```python
from build123d import *

# Parameters (mm, degrees)
ESBO_O4_R                = 3.5
ESBO_O4_R_2              = 1.5
RESSALTO_EXTRUS_O1_DEPTH = 3


with BuildPart() as part:
    # Esboço4 → Ressalto-extrusão1 (new body)
    with BuildSketch(Plane(origin=(0, 0, 0), x_dir=(1, 0, 0), z_dir=(0, 1, 0))):
        with BuildLine():
            Line((-11.987372598, 93.966613318), (-11.987372598, 71.466613318))
            Line((-11.987372598, 71.466613318), (-11.987372598, -8.633386682))
            ThreePointArc((-11.987372598, -8.633386682), (0.012627402, -20.633386682), (12.012627402, -8.633386682))
            Line((12.012627402, -8.633386682), (12.012627402, 71.466613318))
            Line((12.012627402, 71.466613318), (12.012627402, 93.966613318))
            ThreePointArc((12.012627402, 93.966613318), (9.083695214, 101.03768113), (2.012627402, 103.966613318))
            Line((2.012627402, 103.966613318), (0.012627402, 103.966613318))
            Line((0.012627402, 103.966613318), (-1.987372598, 103.966613318))
            ThreePointArc((-1.987372598, 103.966613318), (-9.05844041, 101.03768113), (-11.987372598, 93.966613318))
        make_face()
        Polygon((0.512627402, -17.633386682), (0.012627402, -17.633386682), (-0.487372598, -17.633386682), (-0.487372598, -11.633386682), (0.512627402, -11.633386682), align=None, mode=Mode.SUBTRACT)
        with Locations(Location((0.012627402, -2.633386682, 0), (0, 0, 270))):
            Circle(ESBO_O4_R, mode=Mode.SUBTRACT)
        Polygon((0.012627402, 12.366613318), (0.512627402, 12.366613318), (0.512627402, 6.366613318), (-0.487372598, 6.366613318), (-0.487372598, 12.366613318), align=None, mode=Mode.SUBTRACT)
        with Locations(Location((0.012627402, 67.966742295, 0), (0, 0, 270))):
            Circle(ESBO_O4_R_2, mode=Mode.SUBTRACT)
        Polygon((6.012627402, 94.466613318), (6.012627402, 71.466613318), (2.487372598, 71.466613318), (-2.487372598, 71.466613318), (-5.987372598, 71.466613318), (-5.987372598, 82.966613318), (-5.987372598, 94.466613318), (-2.5, 94.466613318), (2.5, 94.466613318), align=None, mode=Mode.SUBTRACT)
        with Locations(Location((0.012627402, 97.966613318, 0), (0, 0, 270))):
            Circle(ESBO_O4_R_2, mode=Mode.SUBTRACT)
    extrude(amount=RESSALTO_EXTRUS_O1_DEPTH)


solid = part.part
```
The model under review builds one solid part; all positions refer to its coordinate system, in mm. A direction names the side the tool comes from. Give positions to 0.01 mm unless a question says otherwise; leave off trailing zeros. Write each loop counter-clockwise with the first axis right and the second up, starting at its lowest first coordinate (ties: lowest second). Pieces come first, ordered by that corner, then holes. Notation, with made-up numbers: (-15.5, 44.25) -> (-7.5, 44.25) arc R20 ccw to (-7.5, 70.25) -> close; hole circle Ø1 at (89, 51). An arc over 180 degrees is marked (long way). Put each result on its own line as item: value.
(1) We need section C-C, the plane z = -81. Give the boundary of the cut face in (x, y).
Results are:
outline: (-11.99, 0) -> (-5.99, 0) -> (-5.99, 3) -> (-11.99, 3) -> close; (6.01, 0) -> (12.01, 0) -> (12.01, 3) -> (6.01, 3) -> close
(2) We need section A-A, the plane z = -9. Give the boundary of the cut face in (x, y).
Results are:
outline: (-11.99, 0) -> (-0.49, 0) -> (-0.49, 3) -> (-11.99, 3) -> close; (0.51, 0) -> (12.01, 0) -> (12.01, 3) -> (0.51, 3) -> close
(3) We need section B-B, the plane y = 2. Give the boundary of the cut face in (x, z), and give its area (3 significant figures).
Results are:
outline: (-11.99, -93.97) arc R10 ccw to (-1.99, -103.97) -> (2.01, -103.97) arc R10 ccw to (12.01, -93.97) -> (12.01, 8.63) arc R12 ccw to (-11.99, 8.63) -> close; hole (-5.99, -94.47) -> (6.01, -94.47) -> (6.01, -71.47) -> (-5.99, -71.47) -> close; hole circle Ø7 at (0.01, 2.63); hole circle Ø3 at (0.01, -97.97); hole circle Ø3 at (0.01, -67.97); hole (-0.49, -12.37) -> (0.51, -12.37) -> (0.51, -6.37) -> (-0.49, -6.37) -> close; hole (-0.49, 11.63) -> (0.51, 11.63) -> (0.51, 17.63) -> (-0.49, 17.63) -> close
area: 2,550 mm²
(4) For pin 1 Ø6.5 at (x, z) = (0.01, 2.63) entering from +Y; pin 2 Ø1.5 at (y, z) = (1, 14) entering from -X; pin 3 Ø0.9 at (y, z) = (1, 13) entering from +X; pin 4 Ø1 at (x, y) = (-7.5, 2.5) entering from -Z, all flat-tipped, find the tip position at first contact; note any pin that passes through.
Results are:
pin 1: through
pin 2: x = -11.06
pin 3: x = 11.36
pin 4: z = -102.62
(5) We need section D-D, the plane x = 7.25. Give the boundary of the cut face in (y, z).
Results are:
outline: (0, -102.49) -> (3, -102.49) -> (3, 18.21) -> (0, 18.21) -> close
(6) The part is to be moulded in two halves that separate along Z. For faces 3 (the flat face through (0.513, 1, 15)), 4 (the flat face through (0, 0, -43)), 5 (the cylindrical face through (9.16, 1.48, -100.96)), say which applies: pulls with the +Z half, pulls with the -Z half, needs draft (parallel to the pull), parting line crosses it, or undercut.
Results are:
face 3: undercut
face 4: needs draft
face 5: pulls with the -Z half
(7) To check wall thickness, follow probe 1 along X at (y, z) = (2.2, -86); probe 2 along Z at (x, y) = (-2.5, 0.55); probe 3 along Z at (x, y) = (-2, 2.45). State the ranges of each line that lie inside material, in increasing order. Write a range as from..to.
Results are:
probe 1: -11.99..-5.99, 6.01..12.01
probe 2: -103.95..-94.47, -71.47..0.2, 5.07..20.37
probe 3: -103.97..-94.47, -71.47..-0.23, 5.5..20.46
(8) Tool access review of faces 1 (the flat face through (12.013, 1, -42)), 2 (the flat face through (-0.487, 1, 15)): name each direction out of +Z, -Z, +X, -X, +Y, -Y from which nothing blocks a thin tool from reaching the whole face with its end or side.
Results are:
face 1: +Z, -Z, +X, +Y, -Y
face 2: +Y, -Y
